```python
from build123d import *

# Parameters (mm, degrees)
F1_DEPTH = 6.35
F3_DEPTH = 6.351
F5_DEPTH = 6.351


with BuildPart() as f1:
    # F0 (on Top) → F1 (new body)
    with BuildSketch(Plane.XY):
        with BuildLine():
            Line((113.9825, 84.1375), (-113.9825, 84.1375))
            ThreePointArc((-113.9825, 84.1375), (-117.574602, 82.649602), (-119.0625, 79.0575))
            Line((-119.0625, 79.0575), (-119.0625, -79.0575))
            ThreePointArc((-119.0625, -79.0575), (-117.574602, -82.649602), (-113.9825, -84.1375))
            Line((-113.9825, -84.1375), (113.9825, -84.1375))
            ThreePointArc((113.9825, -84.1375), (117.574602, -82.649602), (119.0625, -79.0575))
            Line((119.0625, -79.0575), (119.0625, 79.0575))
            ThreePointArc((119.0625, 79.0575), (117.574602, 82.649602), (113.9825, 84.1375))
        make_face()
    extrude(amount=F1_DEPTH)

    # F2 (on face) → F3 (cut, through all)
    with BuildSketch(Plane.XY.offset(6.35)):
        Polygon((-87.3125, 22.479), (-87.3125, 0), (-87.3125, -22.479), (47.5615, -22.479), (47.5615, -44.901281), (92.462781, 0), (47.5615, 44.901281), (47.5615, 22.479), align=None)
    extrude(amount=-F3_DEPTH, mode=Mode.SUBTRACT)

    # F4 (on face) → F5 (cut, through all)
    with BuildSketch(Plane.XY.offset(6.35)):
        with BuildLine():
            Line((-88.5825, 22.9616), (-88.5825, -22.9616))
            ThreePointArc((-88.5825, -22.9616), (-88.351876, -23.518376), (-87.7951, -23.749))
            Line((-87.7951, -23.749), (45.5041, -23.749))
            ThreePointArc((45.5041, -23.749), (46.060876, -23.979624), (46.2915, -24.5364))
            Line((46.2915, -24.5364), (46.2915, -46.06638))
            ThreePointArc((46.2915, -46.06638), (46.777575, -46.793843), (47.635676, -46.623156))
            Line((47.635676, -46.623156), (93.702056, -0.556776))
            ThreePointArc((93.702056, -0.556776), (93.93268, 0), (93.702056, 0.556776))
            Line((93.702056, 0.556776), (47.635676, 46.623156))
            ThreePointArc((47.635676, 46.623156), (46.777575, 46.793843), (46.2915, 46.06638))
            Line((46.2915, 46.06638), (46.2915, 24.5364))
            ThreePointArc((46.2915, 24.5364), (46.060876, 23.979624), (45.5041, 23.749))
            Line((45.5041, 23.749), (-87.7951, 23.749))
            ThreePointArc((-87.7951, 23.749), (-88.351876, 23.518376), (-88.5825, 22.9616))
        make_face()
    extrude(amount=-F5_DEPTH, mode=Mode.SUBTRACT)


solid = f1.part
```
The listing builds one solid part. Answer for the finished solid, in the listing's coordinates (mm). A direction names the side the tool comes from. Give positions to 0.01 mm unless a question says otherwise; leave off trailing zeros. Order: outer loops, then holes, each group sorted by start corner. A loop starts at its lowest first (then second) coordinate and runs counter-clockwise, first axis right, second up. Notation, with made-up numbers: (79, 63) -> (135, 63) arc R8 cw to (135, 68) -> close; hole circle Ø4 at (-8, -3.5). An arc over 180 degrees is marked (long way). One line per item, written item: value.
1) A tool of negligible diameter and unlimited length cuts with its end or side. For faces 1 (the flat face through (46.292, 35, 3)), 2 (the flat face through (-119.062, 1, 3)), from which of +Z, -Z, +X, -X, +Y, -Y can it reach the whole face along a straight path? Write none if from no direction.
Reported:
face 1: +Z, -Z
face 2: +Z, -Z, -X, +Y, -Y
2) Find section A-A, the plane x = -23. Determine the outline of the cut face in (y, z), plus the area to 3 significant figures.
Reported:
outline: (-84.14, 0) -> (-23.75, 0) -> (-23.75, 6.35) -> (-84.14, 6.35) -> close; (23.75, 0) -> (84.14, 0) -> (84.14, 6.35) -> (23.75, 6.35) -> close
area: 767 mm^2
3) Find section B-B, the plane y = 40. Determine the outline of the cut face in (x, z), plus the area to 3 significant figures.
Reported:
outline: (-119.06, 0) -> (46.29, 0) -> (46.29, 6.35) -> (-119.06, 6.35) -> close; (54.26, 0) -> (119.06, 0) -> (119.06, 6.35) -> (54.26, 6.35) -> close
area: 1,460 mm^2
4) Find section C-C, the plane z = 2. Determine the outline of the cut face in (x, y).
Reported:
outline: (-119.06, -79.06) arc R5.08 ccw to (-113.98, -84.14) -> (113.98, -84.14) arc R5.08 ccw to (119.06, -79.06) -> (119.06, 79.06) arc R5.08 ccw to (113.98, 84.14) -> (-113.98, 84.14) arc R5.08 ccw to (-119.06, 79.06) -> close; hole (-88.58, -22.96) arc R0.79 ccw to (-87.8, -23.75) -> (45.5, -23.75) arc R0.79 cw to (46.29, -24.54) -> (46.29, -46.07) arc R0.79 ccw to (47.64, -46.62) -> (93.7, -0.56) arc R0.79 ccw to (93.7, 0.56) -> (47.64, 46.62) arc R0.79 ccw to (46.29, 46.07) -> (46.29, 24.54) arc R0.79 cw to (45.5, 23.75) -> (-87.8, 23.75) arc R0.79 ccw to (-88.58, 22.96) -> close
5) A flat-ended cylindrical pin translates along its axis: P1, Ø1.5, axis at x = -83, y = 41.5, coming from the -Z side. Find the tip coordinate at first contact, or state that the pin passes through.
Reported:
P1: stops at z = 0
6) Find the intervals of material crossed by line 1 (Y direction, x = -3, z = 1.5); line 2 (X direction, y = -16.5, z = 2.75); line 3 (X direction, y = -14.5, z = 6.25), in increasing order.
Reported:
line 1: y = -84.14 to -23.75, 23.75 to 84.14
line 2: x = -119.06 to -88.58, 77.76 to 119.06
line 3: x = -119.06 to -88.58, 79.76 to 119.06
7) Determine the mould class of faces 3 (the flat face through (119.062, -1, 3)), 4 (the flat face through (46.292, -35, 3)), 5 (the flat face through (2, 84.138, 3)) for opening direction X: pulls with the +X half, pulls with the -X half, needs draft (parallel to the pull), parting line crosses it, or undercut.
Reported:
face 3: pulls with the +X half
face 4: undercut
face 5: needs draft
